Autodesk Inventor part; units mm, degrees
ref_plane "Work Plane4" through (15.7, 23.5, 45) normal (0, -1, 0) x (1, 0, 0)
ref_plane "YZ Plane" through (0, 0, 0) normal (1, 0, 0) x (0, 1, 0)
ref_plane "XZ Plane" through (0, 0, 0) normal (0, 1, 0) x (-1, 0, 0)
sketch "Sketch1" plane through (0, 0, 0) normal (0, 1, 0) x (-1, 0, 0)
  line L0 (-25, 25) -> (25, 25)
  line L1 (25, 25) -> (25, -25)
  line L2 (25, -25) -> (-25, -25)
  line L3 (-25, -25) -> (-25, 25)
  line L4 (-25, 25) -> (25, -25) construction
  line L5 (25, 25) -> (-25, -25) construction
  point P0 (0, 0)
  dimension "d0" = 50
  dimension "d1" = 50
extrude "Extrusion1" add sketch "Sketch1" along normal blind 36.5
sketch "Sketch2" plane through (-25, 0, 25) normal (0, 0, 1) x (1, 0, 0)
  line L0 (0, 0) -> (50, 0)
  line L1 (50, 0) -> (50, 36.5)
  line L2 (0, 36.5) -> (50, 36.5)
  line L3 (0, 0) -> (0, 36.5)
  circle A0 centre (40.7, 23.5) radius 6
  line L4 (25, 0) -> (25, 36.5) construction
  dimension "d4" = 15.7
  dimension "d5" = 13
  dimension "d6" = 12
extrude "Extrusion2" add sketch "Sketch2" along normal blind 20 contours A0
sketch "Sketch4" plane through (0, 36.5, 0) normal (0, 1, 0) x (1, 0, 0)
  circle A0 centre (0, 0) radius 19.25
  dimension "d12" = 38.5
extrude "Extrusion4" add sketch "Sketch4" along normal blind 35
sketch "Sketch7" plane through (25, 0, -25) normal (0, 0, -1) x (-1, 0, 0)
  line L0 (0, 0) -> (50, 0)
  line L1 (50, 0) -> (50, 36.5)
  line L2 (0, 36.5) -> (50, 36.5)
  line L3 (0, 0) -> (0, 36.5)
  line L4 (12.5, 22.5) -> (37.5, 22.5) construction
  point P0 (25, 0)
  point P1 (25, 22.5)
  point P2 (25, 0)
  dimension "d22" = 25
  dimension "d23" = 22.5
hole "Hole2" at (12.5, 22.5, -25) at (-12.5, 22.5, -25) direction (0, 0, 1) diameter 4.134 depth 8
sketch "Sketch9" plane through (-25, 0, -25) normal (-1, 0, 0) x (0, 0, 1)
  line L0 (0, 0) -> (50, 0)
  line L1 (50, 0) -> (50, 36.5)
  line L2 (0, 36.5) -> (50, 36.5)
  line L3 (0, 0) -> (0, 36.5)
  line L4 (12.5, 22.5) -> (37.5, 22.5) construction
  point P0 (25, 0)
  point P1 (25, 22.5)
  point P2 (25, 0)
  dimension "d38" = 25
  dimension "d39" = 22.5
hole "Hole3" at (-25, 22.5, -12.5) at (-25, 22.5, 12.5) direction (1, 0, 0) diameter 4.134 depth 8
chamfer "Chamfer1" distance 0.5 angle 45 4 edges at (25, 18.25, 25) (-25, 18.25, 25) (25, 18.25, -25) (-25, 18.25, -25)
sketch "Sketch10" plane through (15.7, 23.5, 45) normal (0, 0, 1) x (1, 0, 0)
  circle A0 centre (0, 0) radius 6
  point P0 (-15.7, -23.5)
ref_plane "Work Plane4" through (15.7, 23.5, 45) normal (0, -1, 0) x (1, 0, 0)
properties part number "RE38S-600Z-1M-no-end" material "ABS Plastic"
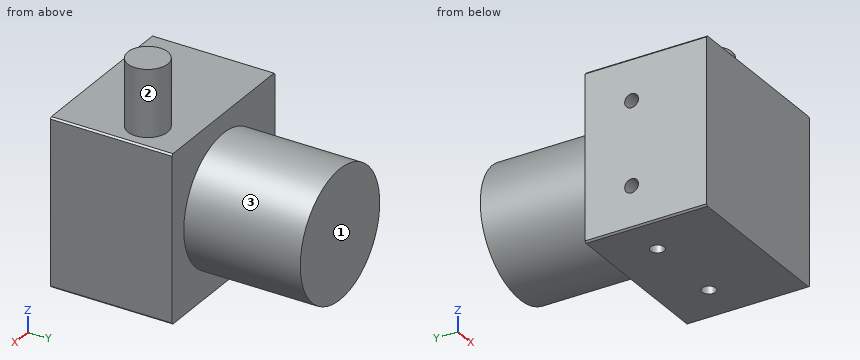
Here's how the part is built. I have some questions about the finished solid (model axes, mm). Face numbers are marked on the shaded views. A direction names the side the tool comes from. Round coordinates to 2 decimals unless told otherwise and drop trailing zeros. Order: outer loops, then holes, each group sorted by start corner. A loop starts at its lowest first (then second) coordinate and runs counter-clockwise, first axis right, second up. Notation, with made-up numbers: (13.25, 86) -> (54.25, 86) arc R17 cw to (54.25, 118) -> close; hole circle Ø8 at (65.5, -7.75). An arc over 180 degrees is marked (long way). Use a Markdown table: item, result. Add a question column.
(1) For pin 1 Ø3.5 at (y, z) = (22.5, 12.5) entering from -X; pin 2 Ø10 at (x, z) = (17.5, 24.5) entering from +Y; pin 3 Ø8 at (x, y) = (-8.5, 16.5) entering from +Z, each with a flat end and sliding along its axis, tell me the tip position at first contact or that it passes through.
(2) Suppose I cut it at C-C, the plane x = 12.5. Please give me the cut outline in (y, z), and give its area (3 significant figures).
(3) Suppose I cut it at A-A, the plane y = 34. Please give me the cut outline in (x, z).
(4) I need wall thicknesses on line 1 along X through (y, z) = (22.5, -18.75); line 2 along Y through (x, z) = (-12.5, -20.25). Which ranges of each line are inside material? Lowest first, please.
(5) Suppose I cut it at D-D, the plane y = 21.5. Please give me the cut outline in (x, z).
(6) Suppose I cut it at B-B, the plane z = 0. Please give me the cut outline in (x, y), and give its area (3 significant figures).
(7) For the marked faces 1, 2 and 3, which set-ups out of +Z, -Z, +X, -X, +Y, -Y let a thin tool reach every point of the face, with its end or its side?
Verdict:
| question | item | result |
|---|---|---|
| 1 | pin 1 | x = -17 |
| 1 | pin 2 | y = 36.5 |
| 1 | pin 3 | z = 25 |
| 2 | outline | (0, -25) -> (20.43, -25) -> (20.43, -17) -> (24.57, -17) -> (24.57, -25) -> (36.5, -25) -> (36.5, -14.64) -> (71.5, -14.64) -> (71.5, 14.64) -> (36.5, 14.64) -> (36.5, 25) -> (28.58, 25) -> (28.58, 45) -> (18.42, 45) -> (18.42, 25) -> (0, 25) -> close |
| 2 | area | 3,020 mm2 |
| 3 | outline | (-25, -24.5) -> (-24.5, -25) -> (24.5, -25) -> (25, -24.5) -> (25, 24.5) -> (24.5, 25) -> (-24.5, 25) -> (-25, 24.5) -> close |
| 4 | line 1 | -25 to -14.57, -10.43 to 10.43, 14.57 to 25 |
| 4 | line 2 | 0 to 20.43, 24.57 to 36.5 |
| 5 | outline | (-25, -24.5) -> (-24.5, -25) -> (-14.31, -25) -> (-14.31, -17) -> (-10.69, -17) -> (-10.69, -25) -> (10.69, -25) -> (10.69, -17) -> (14.31, -17) -> (14.31, -25) -> (24.5, -25) -> (25, -24.5) -> (25, 24.5) -> (24.5, 25) -> (21.36, 25) -> (21.36, 45) -> (10.04, 45) -> (10.04, 25) -> (-24.5, 25) -> (-25, 24.5) -> (-25, 14.31) -> (-17, 14.31) -> (-17, 10.69) -> (-25, 10.69) -> (-25, -10.69) -> (-17, -10.69) -> (-17, -14.31) -> (-25, -14.31) -> close |
| 6 | outline | (-25, 0) -> (25, 0) -> (25, 36.5) -> (19.25, 36.5) -> (19.25, 71.5) -> (-19.25, 71.5) -> (-19.25, 36.5) -> (-25, 36.5) -> close |
| 6 | area | 3,170 mm2 |
| 7 | face 1 | +Z, -Z, +X, -X, +Y |
| 7 | face 2 | +Z |
| 7 | face 3 | +Y |
